Source: CAD feature listing. Evaluate the final solid. Frame: model axes, mm. A direction names the side the tool comes from. Coordinates: 2 decimals unless noted, no trailing zeros. Loops run counter-clockwise (first coordinate to the right, second up) from the corner with the lowest first, then second, coordinate; pieces in that order, holes last.
Item 1: Section query D-D, the plane x = 21.5. Return the cut outline in (y, z), then the cut area to 3 significant figures.
Item 2: Line query: probe 1 along Y at (x, z) = (38, 0.5); probe 2 along Z at (x, y) = (6.5, 16); probe 3 along X at (y, z) = (3.5, 1). Output: solid intervals per line, ascending.
Item 3: Section query C-C, the plane y = 20.5. Return the cut outline in (x, z).
Item 4: Pin query (flat end, axial travel): pin 1 Ø1.2 at (x, z) = (47, 3) entering from -Y; pin 2 Ø2.5 at (y, z) = (20.5, 3.5) entering from -X; pin 3 Ø3 at (x, z) = (41, 1) entering from +Y. Return the tip coordinate at first contact, or that it passes through.
Item 5: Pull-direction query (Y, two-part tool) for faces 5 (the flat face through (48, 23, 4.25)), 6 (the flat face through (1, 25.25, 2)), 7 (the flat face through (24, 0, 1)), 8 (the flat face through (43, 1.25, 1)); classes: +Y half, -Y half, draft (parallel to the pull), parting line (faces both ways), or undercut.
Item 6: Reachability of faces 1 (the flat face through (47, 24, 3)), 2 (the flat face through (48, 19, 3)), 3 (the flat face through (24, 24, 1)), 4 (the flat face through (5, 1.25, 1)) from +Z, -Z, +X, -X, +Y, -Y: full face, straight path, thin tool, end or side. Return the list, or none.
Item 7: Section query B-B, the plane x = 39.5. Return the cut outline in (y, z).
Item 8: Section query A-A, the plane z = 3.75. Return the cut outline in (x, y).
```python
from build123d import *

# Parameters (mm, degrees)
SKETCH1_W           = 50.5
SKETCH1_H           = 24
BOSS_EXTRUDE1_DEPTH = 1.25
SKETCH2_W           = 1.25
SKETCH2_H           = 3
BOSS_EXTRUDE2_DEPTH = 5
SKETCH3_W           = 13
SKETCH3_H           = 3
CUT_EXTRUDE1_DEPTH  = 1.25
SKETCH5_W           = 4.628536498
SKETCH5_H           = 4.25
BOSS_EXTRUDE3_DEPTH = 1.25
SKETCH9_W           = 24.5
SKETCH9_H           = 3
BOSS_EXTRUDE5_DEPTH = 5


with BuildPart() as part:
    # Sketch1 → Boss-Extrude1 (new body)
    with BuildSketch(Plane.XY):
        with Locations((24, 12)):
            Rectangle(SKETCH1_W, SKETCH1_H)
    extrude(amount=BOSS_EXTRUDE1_DEPTH)

    # Sketch2 → Boss-Extrude2 (add)
    with BuildSketch(Plane(origin=(0, 24, 0), x_dir=(1, 0, 0), z_dir=(0, 1, 0))):
        with Locations((47.996463502, -2.75)):
            Rectangle(SKETCH2_W, SKETCH2_H)
        with Locations((45.246463502, -2.75)):
            Rectangle(SKETCH2_W, SKETCH2_H)
        with Locations((2.753536498, -2.75)):
            Rectangle(SKETCH2_W, SKETCH2_H)
        with Locations((0.003536498, -2.75)):
            Rectangle(SKETCH2_W, SKETCH2_H)
    extrude(amount=-BOSS_EXTRUDE2_DEPTH)

    # Sketch3 → Cut-Extrude1 (cut)
    with BuildSketch(Plane(origin=(0, 0, 0), x_dir=(-1, 0, 0), z_dir=(0, 0, -1))):
        with Locations((-42.75, 2.75)):
            Rectangle(SKETCH3_W, SKETCH3_H)
        with Locations((-5.25, 2.75)):
            Rectangle(SKETCH3_W, SKETCH3_H)
    extrude(amount=-CUT_EXTRUDE1_DEPTH, mode=Mode.SUBTRACT)

    # Sketch5 → Boss-Extrude3 (add)
    with BuildSketch(Plane(origin=(0, 24, 0), x_dir=(1, 0, 0), z_dir=(0, 1, 0))):
        with Locations((1.064268249, -2.125)):
            Rectangle(SKETCH5_W, SKETCH5_H)
        with Locations((46.935731751, -2.125)):
            Rectangle(SKETCH5_W, SKETCH5_H)
    extrude(amount=BOSS_EXTRUDE3_DEPTH)

    # Sketch9 → Boss-Extrude5 (add)
    with BuildSketch(Plane.XY.offset(1.25)):
        with Locations((24, 2.75)):
            Rectangle(SKETCH9_W, SKETCH9_H)
    extrude(amount=BOSS_EXTRUDE5_DEPTH)


solid = part.part
```
Verdict:
1. outline: (0, 0) - (24, 0) - (24, 1.25) - (4.25, 1.25) - (4.25, 6.25) - (1.25, 6.25) - (1.25, 1.25) - (0, 1.25) - close
1. area: 45.0 mm2
2. probe 1: y = 0 to 1.25, 4.25 to 24
2. probe 2: z = 0 to 1.25
2. probe 3: x = 11.75 to 36.25
3. outline: (-1.25, 0) - (49.25, 0) - (49.25, 1.25) - (48.62, 1.25) - (48.62, 4.25) - (47.37, 4.25) - (47.37, 1.25) - (45.87, 1.25) - (45.87, 4.25) - (44.62, 4.25) - (44.62, 1.25) - (3.38, 1.25) - (3.38, 4.25) - (2.13, 4.25) - (2.13, 1.25) - (0.63, 1.25) - (0.63, 4.25) - (-0.62, 4.25) - (-0.62, 1.25) - (-1.25, 1.25) - close
4. pin 1: stops at y = 19
4. pin 2: stops at x = -0.62
4. pin 3: stops at y = 24
5. face 5: draft
5. face 6: +Y half
5. face 7: -Y half
5. face 8: undercut
6. face 1: +Z, -Y
6. face 2: +Z, +X, -X, -Y
6. face 3: +Z, -Z, +Y
6. face 4: +Z, -Z, -X
7. outline: (0, 0) - (1.25, 0) - (1.25, 1.25) - (0, 1.25) - close; (4.25, 0) - (24, 0) - (24, 1.25) - (4.25, 1.25) - close
8. outline: (-1.25, 24) - (-0.62, 24) - (-0.62, 19) - (0.63, 19) - (0.63, 24) - (2.13, 24) - (2.13, 19) - (3.38, 19) - (3.38, 25.25) - (-1.25, 25.25) - close; (11.75, 1.25) - (36.25, 1.25) - (36.25, 4.25) - (11.75, 4.25) - close; (44.62, 19) - (45.87, 19) - (45.87, 24) - (47.37, 24) - (47.37, 19) - (48.62, 19) - (48.62, 24) - (49.25, 24) - (49.25, 25.25) - (44.62, 25.25) - close
